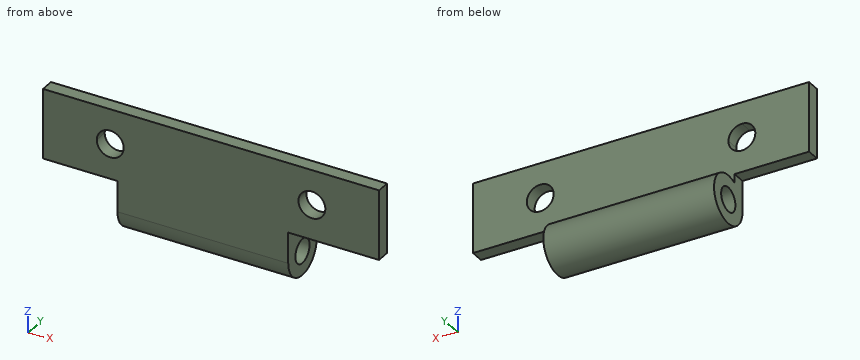
```python
from build123d import *

# Parameters (mm, degrees)
SKETCH1_R               = 0.9
BOSS_EXTRUDE1_DEPTH     = 25
CUT_EXTRUDE1_DEPTH      = 25
CUT_EXTRUDE1_DEPTH_BACK = 25
SKETCH2_W               = 5.541335726
SKETCH2_H               = 4.1
SKETCH2_W_2             = 6.758664274
CUT_EXTRUDE2_DEPTH      = 25
CUT_EXTRUDE2_DEPTH_BACK = 25
SKETCH3_R               = 1


with BuildPart() as part:
    # Sketch1 → Boss-Extrude1 (new body)
    with BuildSketch(Plane(origin=(0, 0, 0), x_dir=(0, 0, -1), z_dir=(1, 0, 0))):
        with BuildLine():
            Line((-6.797691641, -1.201831935), (-14.297691641, -1.201831935))
            Line((-14.297691641, -1.201831935), (-14.297691641, -0.201831935))
            Line((-14.297691641, -0.201831935), (-8.410143191, -0.201831935))
            ThreePointArc((-8.410143191, -0.201831935), (-5.849008343, 2.127873919), (-6.797691641, -1.201831935))
        make_face()
        with Locations((-6.797691641, 0.598168065)):
            Circle(SKETCH1_R, mode=Mode.SUBTRACT)
    extrude(amount=BOSS_EXTRUDE1_DEPTH)

    # Sketch2 → Cut-Extrude1 (cut, two sides: drawn at the far end of the back side and taken through both)
    with BuildSketch(Plane(origin=(0, 0, 0), x_dir=(1, 0, 0), z_dir=(0, 1, 0)).offset(-CUT_EXTRUDE1_DEPTH_BACK)):
        with Locations((2.770667863, -7.047691641)):
            Rectangle(SKETCH2_W, SKETCH2_H)
        with Locations((21.620667863, -7.047691641)):
            Rectangle(SKETCH2_W_2, SKETCH2_H)
    extrude(amount=CUT_EXTRUDE1_DEPTH + CUT_EXTRUDE1_DEPTH_BACK, mode=Mode.SUBTRACT)

    # Sketch3 → Cut-Extrude2 (cut, two sides: drawn at the far end of the back side and taken through both)
    with BuildSketch(Plane(origin=(0, -0.201831935, 0), x_dir=(1, 0, 0), z_dir=(0, 1, 0)).offset(-CUT_EXTRUDE2_DEPTH_BACK)):
        with BuildLine():
            ThreePointArc((4, -11.697691641), (4.292893219, -12.404798422), (5, -12.697691641))
            Line((5, -12.697691641), (5, -11.697691641))
            Line((5, -11.697691641), (4, -11.697691641))
        make_face()
        with BuildLine():
            Line((5, -11.697691641), (5, -12.697691641))
            ThreePointArc((5, -12.697691641), (5.707106781, -12.404798422), (6, -11.697691641))
            ThreePointArc((6, -11.697691641), (5, -10.697691641), (4, -11.697691641))
            Line((4, -11.697691641), (5, -11.697691641))
        make_face()
        with Locations(Location((20, -11.697691641, 0), (0, 0, 90))):
            Circle(SKETCH3_R)
    extrude(amount=CUT_EXTRUDE2_DEPTH + CUT_EXTRUDE2_DEPTH_BACK, mode=Mode.SUBTRACT)


solid = part.part
```
Work out the finished part from the listing and answer in its coordinate system (mm). Coordinates: 2 decimals unless noted, no trailing zeros. Write each loop counter-clockwise with the first axis right and the second up, starting at its lowest first coordinate (ties: lowest second). Pieces come first, ordered by that corner, then holes. Notation, with made-up numbers: (46, -28) - (103, -28) arc R23 cw to (103, 2) - close; hole circle Ø8 at (87.5, -30). An arc over 180 degrees is marked (long way). Answer as a JSON object with one key per item and string values.
Q1. Given pin 1 Ø2 at (y, z) = (-0.5, 7) entering from -X; pin 2 Ø2 at (x, z) = (13, 11.5) entering from +Y, each flat-ended and moving along its own axis, determine where each tip first touches the part or whether it passes through.
Results list:
{"pin 1": "stops at x = 5.54", "pin 2": "stops at y = -0.2"}
Q2. Find section A-A (x = 20). Write down the section's boundary in (y, z).
Results list:
{"outline": "(-1.2, 9.1) - (-0.2, 9.1) - (-0.2, 10.7) - (-1.2, 10.7) - close; (-1.2, 12.7) - (-0.2, 12.7) - (-0.2, 14.3) - (-1.2, 14.3) - close"}
Q3. Find section B-B (y = 0.05). Write down the section's boundary in (x, z).
Results list:
{"outline": "(5.54, 5.08) - (18.24, 5.08) - (18.24, 6.08) - (5.54, 6.08) - close; (5.54, 7.51) - (18.24, 7.51) - (18.24, 8.51) - (5.54, 8.51) - close"}
Q4. Find section D-D (z = 8). Write down the section's boundary in (x, y), plus the area to 3 significant figures.
Results list:
{"outline": "(5.54, -1.2) - (18.24, -1.2) - (18.24, 1.94) - (5.54, 1.94) - close", "area": "39.9 mm^2"}
Q5. Find section C-C (x = 14.5). Write down the section's boundary in (y, z).
Results list:
{"outline": "(-1.2, 6.8) arc R1.8 ccw (long way) to (-0.2, 8.41) - (-0.2, 14.3) - (-1.2, 14.3) - close; hole circle Ø1.8 at (0.6, 6.8)"}
Q6. Consider L1, parallel to Y at x = 14.5, z = 6.75; L2, parallel to X at y = -0.35, z = 12; L3, parallel to X at y = -0.8, z = 9. Determine where each line is inside the solid, lowest interval first. Write a range as from..to.
Results list:
{"L1": "y = -1.2..-0.3, 1.5..2.4", "L2": "x = 0..4.05, 5.95..19.05, 20.95..25", "L3": "x = 5.54..18.24"}
